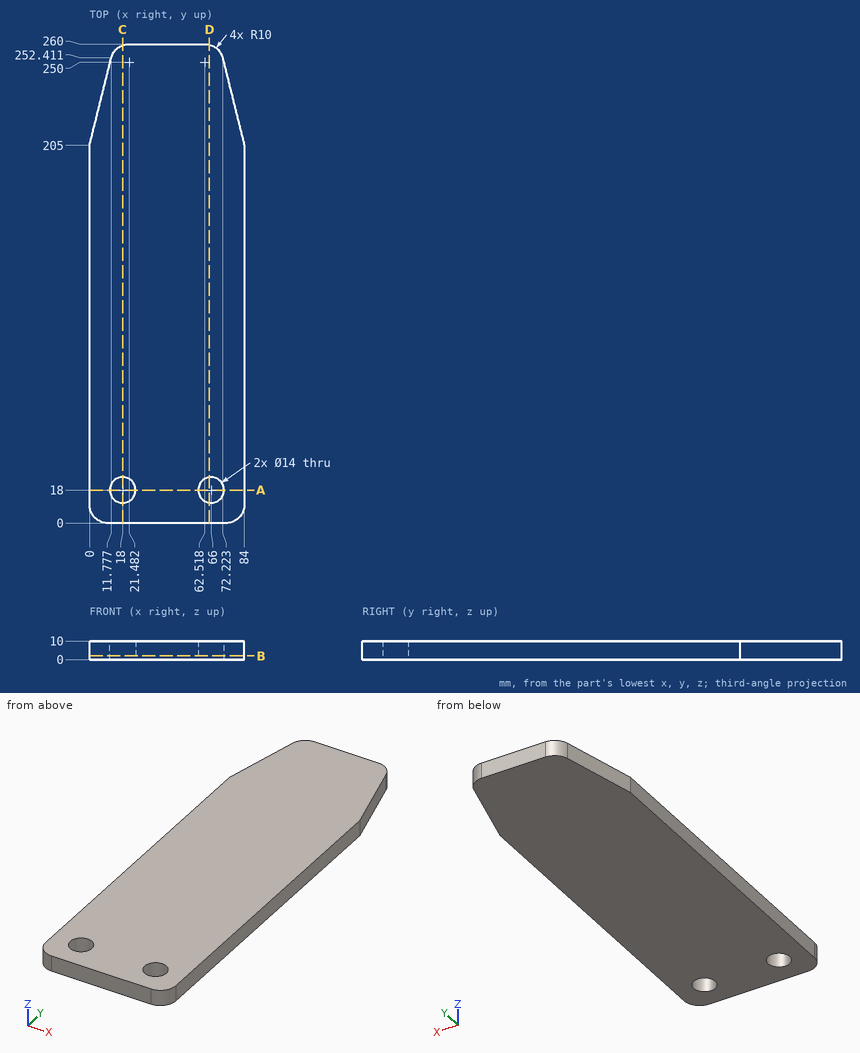
Print and shaded views of the part. All mm, measured from the part's lowest x, y and z. Coordinates: 2 decimals unless noted, no trailing zeros. Order: outer loops, then holes, each group sorted by start corner. A loop starts at its lowest first (then second) coordinate and runs counter-clockwise, first axis right, second up.
(1) Slice it at C-C, the plane x = 18. Write the cut outline in (y, z), and give its area (3 significant figures).
Check sheet entries:
outline: (0, 0) - (11, 0) - (11, 10) - (0, 10) - close; (25, 0) - (259.37, 0) - (259.37, 10) - (25, 10) - close
area: 2,450 mm2
(2) Slice it at D-D, the plane x = 65. Write the cut outline in (y, z).
Check sheet entries:
outline: (0, 0) - (11.07, 0) - (11.07, 10) - (0, 10) - close; (24.93, 0) - (259.69, 0) - (259.69, 10) - (24.93, 10) - close
(3) Probe L1, parallel to Y at x = 18, z = 5 (1 decimal); L2, parallel to Y at x = 64, z = 8; L3, parallel to X at y = 213, z = 6.5. List the from-to ranges inside material, lowest first.
Check sheet entries:
L1: y = 0 to 11, 25 to 259.4
L2: y = 0 to 11.29, 24.71 to 259.89
L3: x = 1.99 to 82.01
(4) Slice it at B-B, the plane z = 2. Write the cut outline in (x, y).
Check sheet entries:
outline: (0, 10) arc R10 ccw to (10, 0) - (74, 0) arc R10 ccw to (84, 10) - (84, 205) - (72.22, 252.41) arc R10 ccw to (62.52, 260) - (21.48, 260) arc R10 ccw to (11.78, 252.41) - (0, 205) - close; hole circle Ø14 at (18, 18); hole circle Ø14 at (66, 18)
(5) Pin check, flat tip, straight feed: pin 1 Ø11 at (x, y) = (66, 18) entering from +Z. Stop position of the tip, or through.
Check sheet entries:
pin 1: passes through
(6) Slice it at A-A, the plane y = 18. Write the cut outline in (x, z).
Check sheet entries:
outline: (0, 0) - (11, 0) - (11, 10) - (0, 10) - close; (25, 0) - (59, 0) - (59, 10) - (25, 10) - close; (73, 0) - (84, 0) - (84, 10) - (73, 10) - close
